Autodesk Inventor part; units mm, degrees
ref_plane "YZ Plane" through (0, 0, 0) normal (1, 0, 0) x (0, 1, 0)
ref_plane "XZ Plane" through (0, 0, 0) normal (0, 1, 0) x (-1, 0, 0)
ref_plane "XY Plane" through (0, 0, 0) normal (0, 0, 1) x (1, 0, 0)
sketch "Szkic1" plane through (0, 0, 0) normal (1, 0, 0) x (0, 1, 0)
  line L0 (29, 29) -> (-29, 29)
  line L1 (-29, 29) -> (-29, -29)
  line L2 (-29, -29) -> (29, -29)
  line L3 (29, -29) -> (29, 29)
  line L4 (28, 28) -> (-28, 28)
  line L5 (-28, 28) -> (-28, -28)
  line L6 (-28, -28) -> (28, -28)
  line L7 (28, -28) -> (28, 28)
  point P0 (0, 0)
  dimension "d0" = 58
  dimension "d1" = 58
  dimension "d2" = 56
  dimension "d3" = 56
extrude "Wyciągnięcie proste1" add sketch "Szkic1" along normal blind 56
sketch "Szkic2" plane through (56, 0, 0) normal (1, 0, 0) x (0, 0, -1)
  line L0 (29, 29) -> (-29, 29)
  line L1 (29, -29) -> (29, 29)
  line L2 (-29, 29) -> (29, 29)
  line L3 (29, 29) -> (29, -29)
  line L4 (29, -29) -> (-29, -29)
  line L5 (-29, -29) -> (-29, 29)
  point P0 (0, 0)
extrude "Wyciągnięcie proste2" add sketch "Szkic2" along normal blind 2
sketch "Szkic3" plane through (0, 0, 0) normal (-1, 0, 0) x (0, 0, 1)
  line L0 (29, 50) -> (-29, 50)
  line L1 (-29, 50) -> (-29, -50)
  line L2 (-29, -50) -> (29, -50)
  line L3 (29, -50) -> (29, 50)
  line L4 (-28, 49) -> (28, 49)
  line L5 (28, 49) -> (28, -49)
  line L6 (28, -49) -> (-28, -49)
  line L7 (-28, -49) -> (-28, 49)
  point P0 (0, 0)
  dimension "d8" = 100
  dimension "d9" = 98
extrude "Wyciągnięcie proste3" add sketch "Szkic3" along normal blind 50
sketch "Szkic4" plane through (0, 0, 0) normal (1, 0, 0) x (0, 0, -1)
  line L0 (-29, 29) -> (-29, 50)
  line L1 (29, -29) -> (29, 29)
  line L2 (-29, 50) -> (29, 50)
  line L3 (29, 50) -> (29, 29)
  line L4 (29, 29) -> (-29, 29)
  line L5 (-29, 29) -> (-29, 50)
  line L6 (29, -50) -> (-29, -50)
  line L7 (-29, -29) -> (29, -29)
  line L8 (29, -29) -> (29, -50)
  line L9 (29, -50) -> (-29, -50)
  line L10 (-29, -50) -> (-29, -29)
  point P0 (0, 0)
extrude "Wyciągnięcie proste4" add sketch "Szkic4" along normal blind 1
sketch "Szkic5" plane through (58, -29, -29) normal (0, 0, -1) x (-1, 0, 0)
  line L0 (108, 78) -> (108, -20)
  line L1 (58, 57) -> (108, 57)
  line L2 (108, 57) -> (108, 0.6199)
  line L3 (108, 0.6199) -> (58, 0.6199)
  line L4 (58, 0.6199) -> (58, 57)
  point P0 (58, 29)
extrude "Wyciągnięcie proste5" cut sketch "Szkic5" against normal blind 1
sketch "Szkic6" plane through (58, -29, -29) normal (0, 0, -1) x (-1, 0, 0)
  line L0 (108, 57) -> (58, 57)
  line L1 (83, 57) -> (83, 78)
  line L2 (58, 78) -> (108, 78)
  line L3 (108, 57) -> (108, 78)
  line L4 (108, 67.5) -> (57, 67.5)
  line L5 (57, 58) -> (57, 79)
  line L6 (58, -20) -> (108, -20)
  line L7 (83, -20) -> (83, 0.6199)
  line L8 (58, 0.6199) -> (108, 0.6199)
  line L9 (58, -20) -> (58, 1)
  line L10 (58, -9.5) -> (108, -9.5)
  line L11 (108, 0.6199) -> (108, -21)
  circle A0 centre (83, 67.5) radius 1.5
  circle A1 centre (83, -9.5) radius 1.5
  point P0 (58, 29)
  dimension "d16" = 3
  dimension "d17" = 3
hole "Otwór1" at (-25, 38.5, -29) at (-25, -38.5, -29) direction (0, 0, 1) diameter 4.9784 depth 1 tip angle 118
sketch "Szkic7" plane through (58, -29, 29) normal (0, 0, 1) x (1, 0, 0)
  line L0 (-57, 79) -> (-57, 58)
  line L1 (-57, 79) -> (0, 79)
  line L2 (0, 58) -> (0, 0)
  line L3 (0, 79) -> (0, 58)
  line L4 (-57, -21) -> (-108, -21)
  line L5 (-57, -21) -> (0, -21)
  line L6 (0, -21) -> (0, 0)
  line L7 (-57, 58) -> (0, 58)
  line L8 (0, 58) -> (-57, 58)
  line L9 (-57, 58) -> (-57, 79)
  line L10 (-57, -21) -> (-57, 0)
  line L11 (-57, 0) -> (0, 0)
  point P0 (-58, 29)
extrude "Wyciągnięcie proste6" add sketch "Szkic7" against normal blind 58
sketch "Szkic8" plane through (58, 50, -29) normal (0, 0, -1) x (-1, 0, 0)
  line L0 (0, 0) -> (108, 0)
  line L1 (108, 0) -> (97, 0)
  line L2 (97, 0) -> (97, -100)
  line L3 (0, -100) -> (108, -100)
  line L4 (108, -100) -> (97, -100)
  line L5 (108, -100) -> (108, 0)
  line L6 (97, 0) -> (108, 0)
  point P0 (58, -50)
  dimension "d27" = 11
extrude "Wyciągnięcie proste7" cut sketch "Szkic8" against normal blind 58
sketch "Szkic9" plane through (58, -50, -29) normal (0, -1, 0) x (1, 0, 0)
  line L0 (0, 58) -> (-97, 58)
  line L1 (-97, 0) -> (-97, 58)
  line L2 (-92.9215, 33.311) -> (-92.9215, 42.811)
  line L3 (0, 0) -> (-97, 0)
  line L4 (-87.1435, 33.311) -> (-97, 33.311)
  line L5 (-87.1435, 33.311) -> (-87.1435, 42.811)
  line L6 (-87.1435, 42.811) -> (-92.9215, 42.811)
  line L7 (-92.9215, 42.811) -> (-92.9215, 33.311)
  line L8 (-97, 0) -> (-48.5, 0)
  line L9 (0, 58) -> (0, 0)
  point P0 (-9.857, 42.811)
  point P1 (-9.857, 33.311)
  point P2 (-4.079, 33.311)
  point P3 (-4.079, 42.811)
  dimension "d54" = 5.778
  dimension "d59" = 5.778
  dimension "d60" = 33.311
  dimension "d61" = 9.5
  dimension "d68" = 4.0785
  dimension "d70" = 9.5
  dimension "d71" = 9.5
  dimension "d72" = 5.778
  dimension "d73" = 5.778
  dimension "d74" = 4.079
  dimension "d75" = 77.2865
  dimension "d76" = 77.2865
hole "Otwór2" at (-29.1435, -50, 4.311) at (-29.1435, -50, 13.811) at (-34.9215, -50, 4.311) at (-34.9215, -50, 13.811) at (48.143, -50, 13.811) at (53.921, -50, 13.811) at (53.921, -50, 4.311) at (48.143, -50, 4.311) direction (0, 1, 0) diameter 3 end through all
sketch "Szkic10" plane through (58, 50, 29) normal (0, 1, 0) x (1, 0, 0)
  line L0 (0, 0) -> (-97, 0)
  line L1 (-58, 1) -> (-97, 1)
  line L2 (0, 58) -> (-97, 58)
  line L3 (-97, 0) -> (-97, 58)
  line L4 (-97, 58) -> (0, 58)
  line L5 (0, 58) -> (0, 0)
  line L6 (-58, 1) -> (-2, 1)
  line L7 (-48.5, 1) -> (-48.5, 58)
  line L8 (-48.5, 58) -> (-53.5, 58)
  line L9 (-53.5, 58) -> (-54.5822, 58)
  line L10 (-48.5, 58) -> (-53.5, 58)
  line L11 (-48.5, 58) -> (-51, 58)
  line L12 (-48.5, 1) -> (-46, 1)
  line L13 (-46, 1) -> (-46, 58)
  line L14 (-46, 1) -> (-46, 0)
  line L15 (-48.5, 1) -> (-48.5, 0)
  line L16 (-48.5, 58) -> (-46, 58)
  line L17 (-46, 0) -> (-42.5, 0)
  line L18 (-42.5, 0) -> (-42.5, 58)
  line L19 (-48.5, 58) -> (-52, 58)
  line L20 (-52, 58) -> (-52, 0)
  line L21 (-48.5, 0) -> (-52, 0)
  line L22 (-52, 58) -> (-52, 52)
  line L23 (-52, 52) -> (-42.5, 52)
  line L24 (-52, 0) -> (-52, 6)
  line L25 (-52, 6) -> (-42.5, 6)
  point P0 (-58, 29)
  point P1 (-46, 6)
  point P2 (-46, 52)
  point P3 (-48.5, 6)
  point P4 (-48.5, 52)
  dimension "d78" = 2.5
  dimension "d79" = 3.5
  dimension "d80" = 3.5
  dimension "d81" = 6
  dimension "d82" = 6
extrude "Wyciągnięcie proste8" cut sketch "Szkic10" against normal blind 17.5 contours L25 L13 L23 L18 | L25 L20 L23 L7
sketch "Szkic11" plane through (15.5, 50, -23) normal (-1, 0, 0) x (0, 0, 1)
  line L0 (0, -17.5) -> (46, -17.5)
  line L1 (46, -17.5) -> (46, -12.5)
  line L2 (46, 0) -> (46, -17.5)
  line L3 (46, -12.5) -> (0, -12.5)
  line L4 (0, 0) -> (0, -17.5)
  line L5 (0, -17.5) -> (46, -17.5)
  line L6 (0, -17.5) -> (0, -12.5)
  line L7 (46, -12.5) -> (46, -17.5)
  point P0 (23, -50)
  dimension "d85" = 5
extrude "Wyciągnięcie proste9" cut sketch "Szkic11" along normal blind 9.75
fillet "Zaokrąglenie1" radius 0.5 2 edges at (9.5, 50, 0) (12, 50, 0)
sketch "Szkic12" plane through (58, -50, -29) normal (0, -1, 0) x (1, 0, 0)
  line L0 (0, 0) -> (-97, 0)
  line L1 (-97, 0) -> (-97, 58)
  line L2 (-97, 58) -> (0, 58)
  line L3 (0, 58) -> (0, 0)
  line L4 (-48.5, 1) -> (-48.5, 58)
  line L5 (-48.5, 58) -> (-53.5, 58)
  line L6 (-53.5, 58) -> (-54.5822, 58)
  line L7 (-48.5, 58) -> (-53.5, 58)
  line L8 (-48.5, 58) -> (-51, 58)
  line L9 (-48.5, 1) -> (-46, 1)
  line L10 (-46, 1) -> (-46, 58)
  line L11 (-46, 1) -> (-46, 0)
  line L12 (-48.5, 1) -> (-48.5, 0)
  line L13 (-48.5, 58) -> (-46, 58)
  line L14 (-46, 0) -> (-42.5, 0)
  line L15 (-42.5, 0) -> (-42.5, 58)
  line L16 (-48.5, 58) -> (-52, 58)
  line L17 (-52, 58) -> (-52, 0)
  line L18 (-48.5, 0) -> (-52, 0)
  line L19 (-52, 58) -> (-52, 52)
  line L20 (-52, 52) -> (-42.5, 52)
  line L21 (-52, 0) -> (-52, 6)
  line L22 (-52, 6) -> (-42.5, 6)
  point P0 (-58, 29)
  point P1 (-46, 6)
  point P2 (-46, 52)
  point P3 (-48.5, 6)
  point P4 (-48.5, 52)
  dimension "d89" = 2.5
  dimension "d90" = 3.5
  dimension "d91" = 3.5
  dimension "d92" = 6
  dimension "d93" = 6
extrude "Wyciągnięcie proste10" cut sketch "Szkic12" against normal blind 10 contours L22 L10 L20 L15 | L22 L17 L20 L4
fillet "Zaokrąglenie2" radius 0.5 2 edges at (12, -50, 0) (9.5, -50, 0)
properties part number "obudowa_silnik_H100_L11_W56"
Geometry check sheet. Reference: the model listing, model coordinates, mm. A direction names the side the tool comes from. Round coordinates to 2 decimals unless told otherwise and drop trailing zeros. Loops run counter-clockwise (first coordinate to the right, second up) from the corner with the lowest first, then second, coordinate; pieces in that order, holes last. Notation, with made-up numbers: (-13.5, -19.75) - (9.5, -19.75) arc R33 cw to (9.5, 13.25) - close; hole circle Ø3 at (70, 8). An arc over 180 degrees is marked (long way). Use a Markdown table: item, result.
Q1. Go/stop test with flat-tipped pins: P1, Ø10, axis at y = -25, z = 14.5, coming from the -X side; P2, Ø3.5, axis at x = -29.14, z = 4.31, coming from the -Y side; P3, Ø2.5, axis at x = -34.92, z = 4.31, coming from the -Y side; P4, Ø8, axis at x = -11, y = 12, coming from the -Z side. Record where each tip stops, or that it passes through.
Solutions:
| item | result |
|---|---|
| P1 | stops at x = 0 |
| P2 | stops at y = -50 |
| P3 | passes through |
| P4 | stops at z = 28 |
Q2. Draft check along Z on faces 5 (the flat face through (28, 0, -28)), 6 (the flat face through (21, 1, -29)), 7 (the flat face through (10.2, 50, 0.4)), 8 (the cylindrical face through (-30.408, 49.507, 3.505)). Enter one of: released by +Z, released by -Z, zero draft, split by the parting line, or undercut.
Solutions:
| item | result |
|---|---|
| face 5 | undercut |
| face 6 | released by -Z |
| face 7 | zero draft |
| face 8 | undercut |
Q3. Cross-section at C-C on x = 26.5. Record the cut outline in (y, z), plus the area to 3 significant figures.
Solutions:
| item | result |
|---|---|
| outline | (-50, -29) - (50, -29) - (50, 29) - (-50, 29) - close; hole (-28, -28) - (28, -28) - (28, 28) - (-28, 28) - close |
| area | 2,660 mm2 |
Q4. Material ranges on line 1 (Y direction, x = -25, z = -28.25); line 2 (X direction, y = 45, z = -2); line 3 (Y direction, x = -20, z = 9.5), recorded low to high.
Solutions:
| item | result |
|---|---|
| line 1 | y = -50 to -40.99, -36.01 to -28.38, 28 to 36.01, 40.99 to 50 |
| line 2 | x = 0 to 6, 9.5 to 12, 15.5 to 58 |
| line 3 | y = -50 to -49, 49 to 50 |
Q5. Cross-section at A-A on x = -25. Record the cut outline in (y, z).
Solutions:
| item | result |
|---|---|
| outline | (-50, -29) - (-40.99, -29) - (-40.99, -28) - (-49, -28) - (-49, 28) - (49, 28) - (49, -28) - (40.99, -28) - (40.99, -29) - (50, -29) - (50, 29) - (-50, 29) - close; (-36.01, -29) - (-28.38, -29) - (-28.38, -28) - (-36.01, -28) - close; (28, -29) - (36.01, -29) - (36.01, -28) - (28, -28) - close |
Q6. Access from +Z, -Z, +X, -X, +Y, -Y to the whole of each face (thin tool, end or side, straight path). Record for faces 1 (the flat face through (11, 32.5, 0)), 2 (the flat face through (28, -28, 0)), 3 (the cylindrical face through (47.129, -38.846, 14.917)), 4 (the flat face through (6, -45, 0)).
Solutions:
| item | result |
|---|---|
| face 1 | none |
| face 2 | -X |
| face 3 | +Y, -Y |
| face 4 | -Y |
Q7. Cross-section at D-D on y = -38.5. Record the cut outline in (x, z).
Solutions:
| item | result |
|---|---|
| outline | (-39, -29) - (-27.49, -29) - (-27.49, -28) - (-39, -28) - close; (-39, 28) - (0, 28) - (0, -28) - (-22.51, -28) - (-22.51, -29) - (58, -29) - (58, 29) - (-39, 29) - close; hole circle Ø3 at (48.14, 4.31); hole circle Ø3 at (48.14, 13.81); hole circle Ø3 at (53.92, 4.31); hole circle Ø3 at (53.92, 13.81) |
